For this review, take the finished solid that the model builds, in its own axes (mm). Face numbers are marked on the shaded views. Give positions to 0.01 mm unless a question says otherwise; leave off trailing zeros. Order: outer loops, then holes, each group sorted by start corner. A loop starts at its lowest first (then second) coordinate and runs counter-clockwise, first axis right, second up. Notation, with made-up numbers: (-9.5, 41) - (44.5, 41) arc R29 cw to (44.5, 67) - close; hole circle Ø11 at (41.25, -24). An arc over 180 degrees is marked (long way). Use a Markdown table: item, result. Add a question column.
1) We need section B-B on z = -5. Write out the cut boundary in (x, y).
2) We need section A-A on x = 0. Write out the cut boundary in (y, z).
3) We need section C-C on y = 22.5. Write out the cut boundary in (x, z).
4) Wall thickness on L1, parallel to Z at x = 0, y = 119; L2, parallel to Z at x = -21, y = 148.5; L3, parallel to X at y = 68, z = 55.5: over which ranges is each line inside the solid? List them lowest first.
5) Clearance check with flat-ended pins moving along their axes: P1, Ø1.5, axis at x = -24.5, y = 47.5, coming from the -Z side; P2, Ø1.5, axis at x = -24.5, y = 43, coming from the +Z side; P3, Ø3, axis at x = 12.5, y = 72.5, coming from the +Z side. State where each tip first meets the part, or that it passes through.
6) Mouldability with a two-part tool opening along Z and no side actions: class the marked faces 1 and 2 as released by +Z, released by -Z, zero draft, split by the parting line, or undercut.
7) We need section D-D on x = 26.5. Write out the cut boundary in (y, z).
Autodesk Inventor part; units mm, degrees
ref_plane "Work Plane1" through (0, 110, -32.8663) normal (-0.7071, 0.7071, 0) x (0, 0, 1)
ref_plane "XZ Plane" through (0, 0, 0) normal (0, 1, 0) x (-1, 0, 0)
ref_plane "XY Plane" through (0, 0, 0) normal (0, 0, 1) x (1, 0, 0)
sketch "Sketch1" plane through (0, 0, 0) normal (0, 1, 0) x (-1, 0, 0)
  circle A0 centre (0, 0) radius 62
  circle A1 centre (0, 0) radius 64
  dimension "d0" = 2
  dimension "d1" = 128
extrude "Extrusion1" add sketch "Sketch1" along normal blind 180
sketch "Sketch2" plane through (0, 0, 0) normal (1, 0, 0) x (0, 1, 0)
  line L0 (20, 58) -> (62, 58)
  line L1 (62, 58) -> (62, -58)
  line L2 (62, -58) -> (20, -58)
  line L3 (20, -58) -> (20, 58)
  line L4 (0, -64) -> (0, 64)
  point P0 (0, 0)
  point P1 (0, 0)
  point P2 (41, 58)
  dimension "d4" = 42
  dimension "d5" = 116
  dimension "d6" = 20
  dimension "d7" = 58
extrude "Extrusion2" cut sketch "Sketch2" against normal through all
sketch "Sketch3" plane through (0, 0, 0) normal (1, 0, 0) x (0, 1, 0)
  line L0 (110, -32.8663) -> (110, 39.5028)
  line L1 (0, -64) -> (0, 64)
  point P0 (0, 0)
  point P1 (110, 3.3182)
  dimension "d10" = 110
ref_plane "Work Plane1" through (0, 110, -32.8663) normal (-0.7071, 0.7071, 0) x (0, 0, 1)
sketch "Sketch4" plane through (0, 110, -32.8663) normal (-0.7071, 0.7071, 0) x (0, 0, 1)
  circle A0 centre (32.8663, -40) radius 35
  line L0 (0, 0) -> (72.3691, 0) construction
  point P0 (32.8663, -77.7817)
  point P1 (36.1845, 0)
  dimension "d12" = 70
  dimension "d15" = 40
extrude "Extrusion3" cut sketch "Sketch4" along normal through all
properties part number "Insulation Shaft"
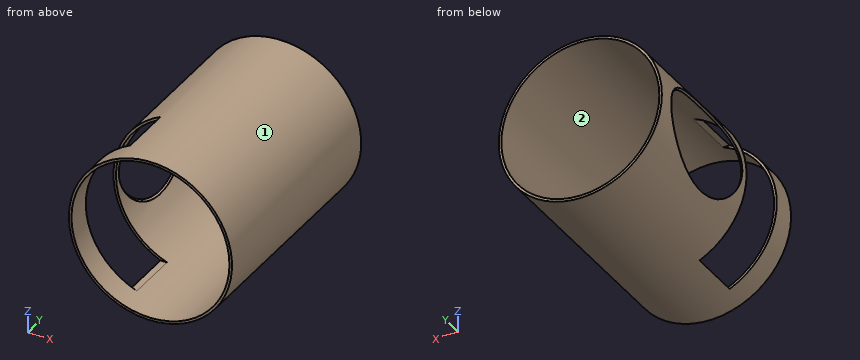
Checked values:
| question | item | result |
|---|---|---|
| 1 | outline | (-63.8, 0) - (-61.8, 0) - (-61.8, 20) - (-63.8, 20) - close; (-63.8, 62) - (-61.8, 62) - (-61.8, 66.24) - (-63.8, 68.25) - close; (-63.8, 166.23) - (-61.8, 164.22) - (-61.8, 180) - (-63.8, 180) - close; (61.8, 0) - (63.8, 0) - (63.8, 180) - (61.8, 180) - close |
| 2 | outline | (0, -64) - (180, -64) - (180, -62) - (0, -62) - close; (0, 62) - (180, 62) - (180, 64) - (0, 64) - close |
| 3 | outline | (-27.06, -58) arc R64 ccw (long way) to (-27.06, 58) - (-21.91, 58) arc R62 cw (long way) to (-21.91, -58) - close |
| 4 | L1 | -64 to -62, 62 to 64 |
| 4 | L2 | -60.46 to -58.34, 58.34 to 60.46 |
| 4 | L3 | -31.87 to -27.64, 27.64 to 31.87 |
| 5 | P1 | z = -59.43 |
| 5 | P2 | z = 59.43 |
| 5 | P3 | z = 63.05 |
| 6 | face 1 | split by the parting line |
| 6 | face 2 | undercut |
| 7 | outline | (0, -58.26) - (180, -58.26) - (180, -56.05) - (0, -56.05) - close; (0, 56.05) - (180, 56.05) - (180, 58.26) - (0, 58.26) - close |
